For this review, take the finished solid that the model builds, in its own axes (mm). A direction names the side the tool comes from. Give positions to 0.01 mm unless a question says otherwise; leave off trailing zeros. Loops run counter-clockwise (first coordinate to the right, second up) from the corner with the lowest first, then second, coordinate; pieces in that order, holes last.
```python
from build123d import *

# Parameters (mm, degrees)
EXTRUDE_1_DEPTH     = 18
SKETCH_2_R          = 10
CUT_EXTRUDE_1_DEPTH = 18
SKETCH_3_R          = 4
EXTRUDE_2_DEPTH     = 30
SKETCH_4_R          = 4
EXTRUDE_3_DEPTH     = 30


with BuildPart() as part:
    # 草图1 → 凸台-拉伸1 (new body)
    with BuildSketch(Plane.XY):
        with BuildLine():
            Line((-0.769230769, -19.985201626), (-130.576923077, -14.988901219))
            ThreePointArc((-130.576923077, -14.988901219), (-145, 0), (-130.576923077, 14.988901219))
            Line((-130.576923077, 14.988901219), (-23.583519409, 19.107079247))
            ThreePointArc((-23.583519409, 19.107079247), (-15.488001892, 21.85715805), (-10.210076964, 28.583512616))
            Line((-10.210076964, 28.583512616), (48.810330778, 177.946063765))
            ThreePointArc((48.810330778, 177.946063765), (67.89099845, 186.528985226), (76.990642321, 167.689269171))
            Line((76.990642321, 167.689269171), (18.973261361, -6.325768991))
            ThreePointArc((18.973261361, -6.325768991), (11.379442316, -16.447136303), (-0.769230769, -19.985201626))
        make_face()
    extrude(amount=EXTRUDE_1_DEPTH)

    # 草图2 → 切除-拉伸1 (cut)
    with BuildSketch(Plane.XY):
        Circle(SKETCH_2_R)
    extrude(amount=CUT_EXTRUDE_1_DEPTH, mode=Mode.SUBTRACT)

    # 草图3 → 凸台-拉伸2 (add)
    with BuildSketch(Plane.XY):
        with Locations((-130, 0)):
            Circle(SKETCH_3_R)
    extrude(amount=-EXTRUDE_2_DEPTH)

    # 草图4 → 凸台-拉伸3 (add)
    with BuildSketch(Plane.XY.offset(18)):
        with Locations(Location((62.7606963, 172.433595914, 0), (0, 0, 180))):
            Circle(SKETCH_4_R)
    extrude(amount=EXTRUDE_3_DEPTH)


solid = part.part
```
Q1. Machinability: for faces 1 (the flat face through (-77.83, 17.02, 8.87)), 2 (the cylindrical face through (-126.305, -1.532, -14.79)), 3 (the cylindrical face through (66.757, 172.258, 32.79)), which of the approach directions +Z, -Z, +X, -X, +Y, -Y give a long, thin tool a straight path to every point of the face, cutting with its end or side? Answer none if there is none.
Answers:
face 1: +Z, -Z, -X, +Y
face 2: -Z
face 3: +Z
Q2. Consider section C-C on y = 148. Give the boundary of the cut face in (x, z).
Answers:
outline: (36.98, 0) - (70.43, 0) - (70.43, 18) - (36.98, 18) - close
Q3. Consider section A-A on y = 0. Give the boundary of the cut face in (x, z).
Answers:
outline: (-145, 0) - (-134, 0) - (-134, -30) - (-126, -30) - (-126, 0) - (-10, 0) - (-10, 18) - (-145, 18) - close; (10, 0) - (21.08, 0) - (21.08, 18) - (10, 18) - close
Q4. For probe 1 along Z at (x, y) = (-98, 14); probe 2 along X at (y, z) = (102.5, 3); probe 3 along Y at (x, z) = (64, 42.5), list the stretches that pass through material, from the lowest coordinate up.
Answers:
probe 1: z = 0 to 18
probe 2: x = 19 to 55.26
probe 3: y = 168.63 to 176.24
Q5. For pin 1 Ø5 at (y, z) = (84.5, 0) entering from +X; pin 2 Ø10 at (x, y) = (-89, 12) entering from +Z; pin 3 Ø3 at (x, z) = (15, 6) entering from -Y, all flat-tipped, find the tip position at first contact; note any pin that passes through.
Answers:
pin 1: stops at x = 50.09
pin 2: stops at z = 18
pin 3: stops at y = -14.76
Q6. Consider section B-B on z = -22. Give the boundary of the cut face in (x, y).
Answers:
outline: circle Ø8 at (-130, 0)
Q7. Consider section D-D on x = -32.5. Give the boundary of the cut face in (y, z).
Answers:
outline: (-18.76, 0) - (18.76, 0) - (18.76, 18) - (-18.76, 18) - close
